Autodesk Fusion 360 part; units mm, degrees
sketch "Sketch1" plane through (0, 0, 0) normal (0, 0, 1) x (1, 0, 0)
  line L0 (2.6, 7.5) -> (-2.6, 7.5)
  line L1 (-2.6, 7.5) -> (-2.6, -7.5)
  line L2 (-2.6, -7.5) -> (2.6, -7.5)
  line L3 (2.6, -7.5) -> (2.6, 7.5)
  line L4 (2.6, 7.5) -> (-2.6, -7.5) construction
  line L5 (-2.6, 7.5) -> (2.6, -7.5) construction
  circle A0 centre (0, 0) radius 1.35
  dimension "d1" = 5.2
  dimension "d2" = 15
  dimension "d3" = 2.7
extrude "Extrude1" add sketch "Sketch1" along normal blind 2.3
fillet "Fillet1" radius 0.5 4 edges at (2.6, 7.5, 1.15) (-2.6, 7.5, 1.15) (-2.6, -7.5, 1.15) (2.6, -7.5, 1.15)
Design review of the part built by this model. Coordinates are the model's own, in mm. Coordinates: 2 decimals unless noted, no trailing zeros. Write each loop counter-clockwise with the first axis right and the second up, starting at its lowest first coordinate (ties: lowest second). Pieces come first, ordered by that corner, then holes.
1) Add section A-A (y = 0). Write out the cut boundary in (x, z).
2) Add section B-B (z = 2.15). Write out the cut boundary in (x, y), plus the area to 3 significant figures.
3) Mouldability with a two-part tool opening along X and no side actions: class faces 1 (the cylindrical face through (-0.29, 1.32, 1.13)), 2 (the flat face through (-2.6, 0, 1)), 3 (the flat face through (2.6, 0, 1)), 4 (the flat face through (0, 7.5, 1)) as +X half, -X half, draft (parallel to the pull), parting line (faces both ways), or undercut.
4) To check wall thickness, follow L1, parallel to Y at x = 0, z = 1.5. State the ranges of the line that lie inside material, in increasing order.
5) Add section C-C (x = 0). Write out the cut boundary in (y, z), plus the area to 3 significant figures.
Check result:
1. outline: (-2.6, 0) - (-1.35, 0) - (-1.35, 2.3) - (-2.6, 2.3) - close; (1.35, 0) - (2.6, 0) - (2.6, 2.3) - (1.35, 2.3) - close
2. outline: (-2.6, -7) arc R0.5 ccw to (-2.1, -7.5) - (2.1, -7.5) arc R0.5 ccw to (2.6, -7) - (2.6, 7) arc R0.5 ccw to (2.1, 7.5) - (-2.1, 7.5) arc R0.5 ccw to (-2.6, 7) - close; hole circle Ø2.7 at (0, 0)
2. area: 72.1 mm2
3. face 1: undercut
3. face 2: -X half
3. face 3: +X half
3. face 4: draft
4. L1: y = -7.5 to -1.35, 1.35 to 7.5
5. outline: (-7.5, 0) - (-1.35, 0) - (-1.35, 2.3) - (-7.5, 2.3) - close; (1.35, 0) - (7.5, 0) - (7.5, 2.3) - (1.35, 2.3) - close
5. area: 28.3 mm2
